Answer from the drawing. Dimensions are ordinates in mm from the lowest x, y and z of the part. Round coordinates to 2 decimals unless told otherwise and drop trailing zeros. Write each loop counter-clockwise with the first axis right and the second up, starting at its lowest first coordinate (ties: lowest second). Pieces come first, ordered by that corner, then holes. Notation, with made-up numbers: (66.5, 67.5) - (76.5, 67.5) arc R21 ccw to (76.5, 91.5) - close; hole circle Ø5 at (17, -32). An arc over 180 degrees is marked (long way). Return JSON: item names as keys, results as strings. Group by question number.
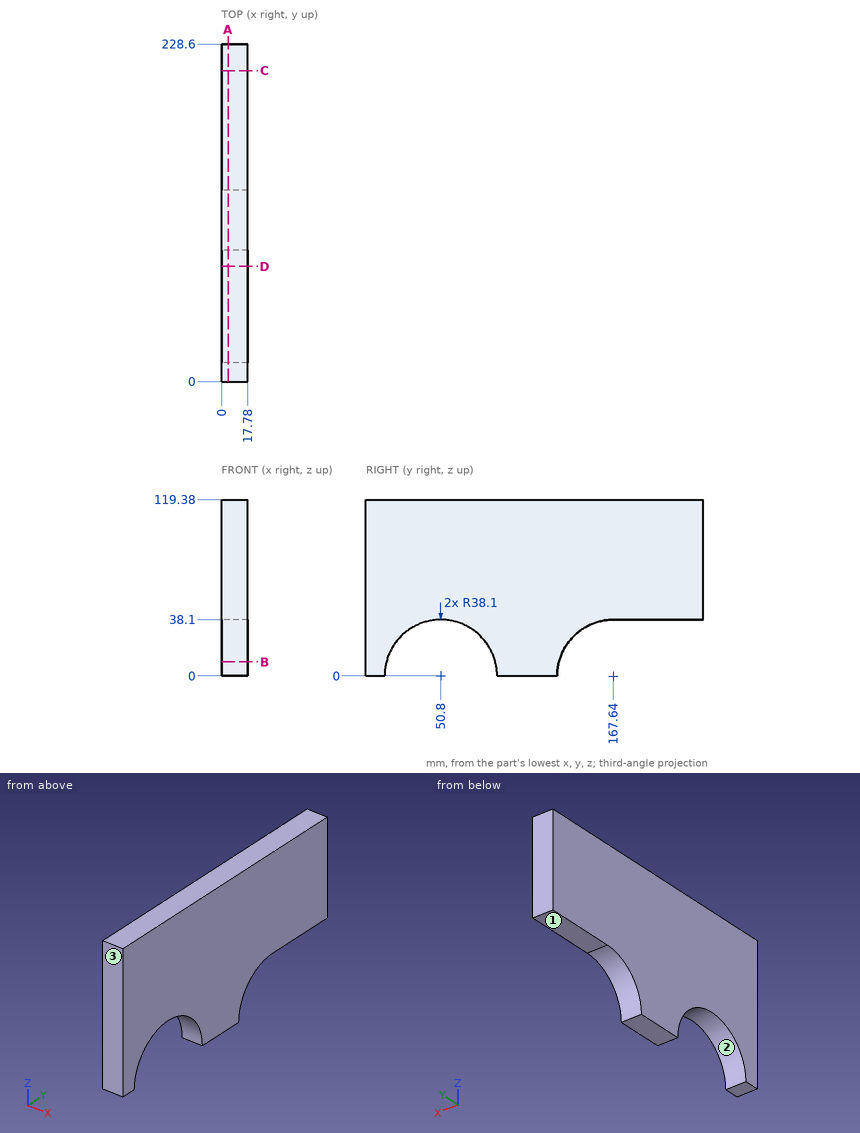
(1) Consider line 1 (Z direction, x = 16.75, y = 209); line 2 (Z direction, x = 12.5, y = 69). Determine where each line is inside the solid, lowest interval first.
(2) Determine the mould class of the marked faces 1, 2 and 3 for opening direction Y: +Y half, -Y half, draft (parallel to the pull), parting line (faces both ways), or undercut.
(3) Find section D-D (y = 78). Write down the section's boundary in (x, z), plus the area to 3 significant figures.
(4) Flat-ended cylindrical pins translate along their axes: pin 1 (4 mm diameter, centred on x = 11.5, y = 204.5, fed in from -Z); pin 2 (10 mm diameter, centred on x = 9.5, y = 52.5, fed in from -Z). Find the tip coordinate at first contact, or state that the pin passes through.
(5) Find section B-B (z = 9.5). Write down the section's boundary in (x, y).
(6) Find section C-C (y = 210.5). Write down the section's boundary in (x, z), plus the area to 3 significant figures.
(7) Find section A-A (x = 4.5). Write down the section's boundary in (y, z), plus the area to 3 significant figures.
Check sheet entries:
{
 "1": {"line 1": "z = 38.1 to 119.38", "line 2": "z = 33.47 to 119.38"},
 "2": {"face 1": "draft", "face 2": "undercut", "face 3": "-Y half"},
 "3": {"outline": "(0, 26.68) - (17.78, 26.68) - (17.78, 119.38) - (0, 119.38) - close", "area": "1,650 mm^2"},
 "4": {"pin 1": "stops at z = 38.1", "pin 2": "stops at z = 37.51"},
 "5": {"outline": "(0, 0) - (17.78, 0) - (17.78, 13.9) - (0, 13.9) - close; (0, 87.7) - (17.78, 87.7) - (17.78, 130.74) - (0, 130.74) - close"},
 "6": {"outline": "(0, 38.1) - (17.78, 38.1) - (17.78, 119.38) - (0, 119.38) - close", "area": "1,450 mm^2"},
 "7": {"outline": "(0, 0) - (12.7, 0) arc R38.1 cw to (88.9, 0) - (129.54, 0) arc R38.1 cw to (167.64, 38.1) - (228.6, 38.1) - (228.6, 119.38) - (0, 119.38) - close", "area": "21,500 mm^2"}
}
